from build123d import *

# Parameters (mm, degrees)
BOSS_EXTRUDE1_DEPTH = 1.016
SKETCH2_R           = 3.175
CUT_EXTRUDE1_DEPTH  = 3.032


with BuildPart() as part:
    # Sketch1 → Boss-Extrude1 (new body, symmetric)
    with BuildSketch(Plane(origin=(0, 0, 0), x_dir=(0, 0, -1), z_dir=(1, 0, 0))):
        with BuildLine():
            Line((-12.382449747, -9.877777778), (-6.191224873, 17.286111111))
            ThreePointArc((-6.191224873, 17.286111111), (0, 22.225), (6.191224873, 17.286111111))
            Line((6.191224873, 17.286111111), (12.382449747, -9.877777778))
            ThreePointArc((12.382449747, -9.877777778), (0, 0), (-12.382449747, -9.877777778))
        make_face()
    extrude(amount=BOSS_EXTRUDE1_DEPTH, both=True)

    # Sketch2 → Cut-Extrude1 (cut, through all)
    with BuildSketch(Plane(origin=(1.016, 0, 0), x_dir=(0, 0, -1), z_dir=(1, 0, 0))):
        with Locations((0, 15.875)):
            Circle(SKETCH2_R)
    extrude(amount=-CUT_EXTRUDE1_DEPTH, mode=Mode.SUBTRACT)


solid = part.part
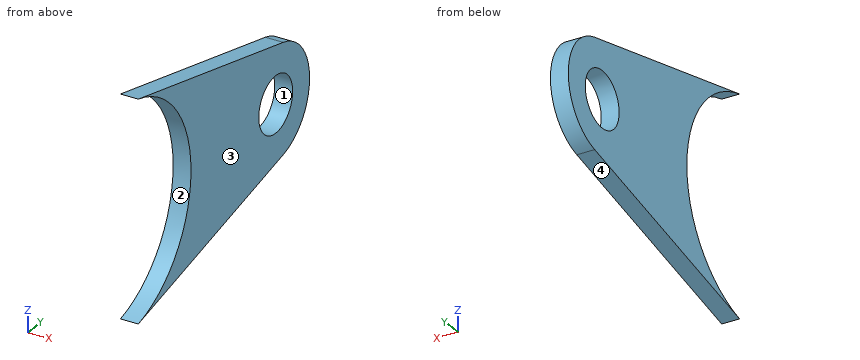
Read the model definition and answer for the solid it produces. Units are mm, in the model's axes. Face numbers are marked on the shaded views. Give positions to 0.01 mm unless a question says otherwise; leave off trailing zeros. Loops run counter-clockwise (first coordinate to the right, second up) from the corner with the lowest first, then second, coordinate; pieces in that order, holes last. Notation, with made-up numbers: (82, -24) -> (134, -24) arc R12 cw to (134, -1) -> close; hole circle Ø6 at (41, 32). An arc over 180 degrees is marked (long way). Answer as CSV lines item,"result".
Item 1: Find section A-A on y = -3.5. Give the vertices of the cut face in (x, z) (3 decimals), plus the area to 3 significant figures.
Returned:
outline,"(-1.016, -10.929) -> (1.016, -10.929) -> (1.016, -8.755) -> (-1.016, -8.755) -> close; (-1.016, 8.755) -> (1.016, 8.755) -> (1.016, 10.929) -> (-1.016, 10.929) -> close"
area,"8.83 mm²"
Item 2: Determine the mould class of the marked faces 1, 2, 3 and 4 for opening direction Z: +Z half, -Z half, draft (parallel to the pull), parting line (faces both ways), or undercut.
Returned:
face 1,"undercut"
face 2,"undercut"
face 3,"draft"
face 4,"-Z half"
Item 3: Find section C-C on x = -0.45. Give the vertices of the cut face in (y, z) (3 decimals).
Returned:
outline,"(-9.878, -12.382) -> (17.286, -6.191) arc R6.35 ccw to (17.286, 6.191) -> (-9.878, 12.382) arc R12.7 cw to start; hole circle Ø6.35 at (15.875, 0)"
Item 4: Consider line 1 (Z direction, x = -0.75, y = -1.5); line 2 (Z direction, x = 0.25, y = -2); line 3 (Z direction, x = 0.15, y = 11). Determine where each line is inside the solid, lowest interval first. Write a range as [from, to].
Returned:
line 1,"z = [-10.47, -5.99], [5.99, 10.47]"
line 2,"z = [-10.59, -6.84], [6.84, 10.59]"
line 3,"z = [-7.62, 7.62]"
Item 5: Find section B-B on z = 0. Give the vertices of the cut face in (x, y) (3 decimals), plus the area to 3 significant figures.
Returned:
outline,"(-1.016, 0) -> (1.016, 0) -> (1.016, 12.7) -> (-1.016, 12.7) -> close; (-1.016, 19.05) -> (1.016, 19.05) -> (1.016, 22.225) -> (-1.016, 22.225) -> close"
area,"32.3 mm²"
Item 6: Find section D-D on z = -4. Give the vertices of the cut face in (x, y).
Returned:
outline,"(-1.02, -0.65) -> (1.02, -0.65) -> (1.02, 20.81) -> (-1.02, 20.81) -> close"
